Could you check a few things on this model? Use its own coordinates, in mm. Face numbers are marked on the shaded views. Coordinates: 2 decimals unless noted, no trailing zeros. Order: outer loops, then holes, each group sorted by start corner. A loop starts at its lowest first (then second) coordinate and runs counter-clockwise, first axis right, second up.
Autodesk Inventor part; units mm, degrees
ref_plane "YZ Plane" through (0, 0, 0) normal (1, 0, 0) x (0, 1, 0)
ref_plane "XZ Plane" through (0, 0, 0) normal (0, 1, 0) x (-1, 0, 0)
ref_plane "XY Plane" through (0, 0, 0) normal (0, 0, 1) x (1, 0, 0)
sketch "Sketch1" plane through (0, 0, 0) normal (0, 0, 1) x (1, 0, 0)
  line L0 (7.9375, 16.002) -> (11.176, 16.002)
  line L1 (11.176, 16.002) -> (11.176, 14.732)
  line L2 (11.176, 14.732) -> (25.4, 14.732)
  line L3 (25.4, 14.732) -> (25.4, 0)
  line L4 (25.4, 0) -> (19.05, 0)
  line L5 (19.05, 0) -> (19.05, 1.27)
  line L6 (19.05, 1.27) -> (7.9375, 1.27)
  line L7 (7.9375, 1.27) -> (7.9375, 16.002)
  line L8 (0, -2.0008) -> (0, 23.5688) construction
  point P0 (0, 0)
  dimension "d0" = 25.4
  dimension "d1" = 19.05
  dimension "d2" = 7.9375
  dimension "d3" = 1.27
  dimension "d4" = 11.176
  dimension "d5" = 16.002
  dimension "d6" = 1.27
revolve "Revolution1" add sketch "Sketch1" angle 360 about axis through (0, -2.0008, 0) along (0, 1, 0)
properties part number "Load Cell"
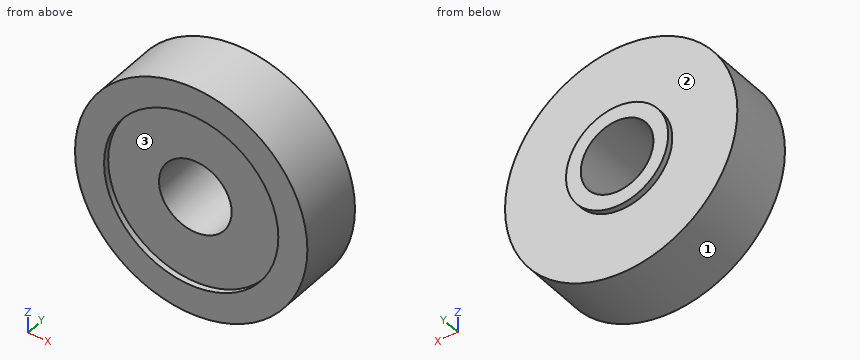
Item 1: Thinking about a two-plate mould opening in X: for the marked faces 1, 2 and 3, which applies, +X half, -X half, draft (parallel to the pull), parting line (faces both ways), or undercut?
Item 2: I need wall thicknesses on line 1 (Z direction, x = 0, y = 0.75); line 2 (Z direction, x = 0, y = 12.25). Which ranges of each line are inside material? Lowest first, please.
Item 3: For pin 1 Ø6 at (x, z) = (11.5, 7.5) entering from -Y; pin 2 Ø1.5 at (y, z) = (14.5, 8.5) entering from +X; pin 3 Ø2 at (y, z) = (6.5, -8.5) entering from -X; pin 4 Ø8 at (x, z) = (-0.5, 14.5) entering from +Y, each with a flat end and sliding along its axis, tell me the tip position at first contact or that it passes through.
Item 4: Suppose I cut it at D-D (z = -16). List the corners of the cut face in (x, y) for me, and give its area (3 significant figures).
Item 5: Suppose I cut it at A-A (x = 0). List the corners of the cut face in (y, z) for me.
Item 6: Suppose I cut it at C-C (y = 9.5). List the corners of the cut face in (x, z) for me (1 decimal).
Item 7: Suppose I cut it at B-B (z = 6). List the corners of the cut face in (x, y) for me, and give its area (3 significant figures).
Geometry results:
1. face 1: parting line
1. face 2: draft
1. face 3: undercut
2. line 1: z = -25.4 to -19.05, 19.05 to 25.4
2. line 2: z = -25.4 to -7.94, 7.94 to 25.4
3. pin 1: stops at y = 1.27
3. pin 2: stops at x = 24.19
3. pin 3: stops at x = -24.27
3. pin 4: stops at y = 16
4. outline: (-19.73, 0) - (-10.34, 0) - (-10.34, 1.27) - (10.34, 1.27) - (10.34, 0) - (19.73, 0) - (19.73, 14.73) - (-19.73, 14.73) - close
4. area: 555 mm2
5. outline: (0, -25.4) - (14.73, -25.4) - (14.73, -11.18) - (16, -11.18) - (16, -7.94) - (1.27, -7.94) - (1.27, -19.05) - (0, -19.05) - close; (0, 19.05) - (1.27, 19.05) - (1.27, 7.94) - (16, 7.94) - (16, 11.18) - (14.73, 11.18) - (14.73, 25.4) - (0, 25.4) - close
6. outline: circle Ø50.8 at (0, 0); hole circle Ø15.9 at (0, 0)
7. outline: (-24.68, 0) - (-18.08, 0) - (-18.08, 1.27) - (-5.2, 1.27) - (-5.2, 16) - (-9.43, 16) - (-9.43, 14.73) - (-24.68, 14.73) - close; (5.2, 1.27) - (18.08, 1.27) - (18.08, 0) - (24.68, 0) - (24.68, 14.73) - (9.43, 14.73) - (9.43, 16) - (5.2, 16) - close
7. area: 552 mm2
